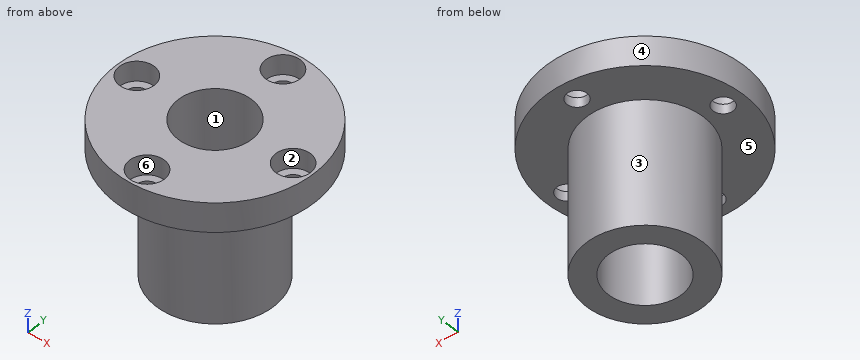
```python
from build123d import *

# Parameters (mm, degrees)
HOLE_WIZARD_1_D           = 5.5
HOLE_WIZARD_1_CBORE_D     = 9.5
HOLE_WIZARD_1_CBORE_DEPTH = 5.4


with BuildPart() as part:
    # 草图1 → 旋转1 (revolve)
    with BuildSketch(Plane(origin=(0, 0, 0), x_dir=(0, 0, 1), z_dir=(0, -1, 0))):
        Polygon((0, 10), (42, 10), (42, 27), (34, 27), (34, 16), (0, 16), align=None)
    revolve(axis=Axis((0, 0, 0), (0, 0, 1)))

    # 孔1 (through all)
    with Locations(Plane.XY.offset(42)):
        with Locations((0, -21.5), (-21.5, 0), (0, 21.5), (21.5, 0)):
            CounterBoreHole(HOLE_WIZARD_1_D / 2, HOLE_WIZARD_1_CBORE_D / 2, HOLE_WIZARD_1_CBORE_DEPTH)


solid = part.part
```
The listing builds one solid part. Answer for the finished solid, in the listing's coordinates (mm). Face numbers are marked on the shaded views. A direction names the side the tool comes from. Coordinates: 2 decimals unless noted, no trailing zeros. Write each loop counter-clockwise with the first axis right and the second up, starting at its lowest first coordinate (ties: lowest second). Pieces come first, ordered by that corner, then holes. Notation, with made-up numbers: M 3.5,-17.75 L 41.5,-17.75 A30 ccw 41.5,14.25 Z; hole C 46,75 d4. An arc over 180 degrees is marked long. Use a Markdown table: item, result. Add a question column.
1. For a pull along X with two mould halves and no side action, classify the marked faces 4, 5 and 6 as +X half, -X half, draft (parallel to the pull), parting line (faces both ways), or undercut.
2. Section C-C (z = 3) is taken. Give the vertices of the cut face in (x, y).
3. Straight lines are drawn through the part: line 1 along X through (y, z) = (0, 19); line 2 along Y through (x, z) = (0, 35.6); line 3 along Z through (x, y) = (16.5, 13). For each, find the intervals that lie inside material, in ascending order. Write a range as [from, to].
4. Which of the six approach directions +Z, -Z, +X, -X, +Y, -Y give full straight-line access (tool end or side, diameter ignored) to the marked faces 1, 2 and 3?
5. Given P1, Ø7.5, axis at x = 0, y = 23.5, coming from the +Z side; P2, Ø6.5, axis at x = 21.5, y = 0, coming from the -Z side; P3, Ø8, axis at x = -12, z = 14, coming from the -Y side; P4, Ø4, axis at x = -21, z = 33, coming from the -Y side, each flat-ended and moving along its own axis, determine where each tip first touches the part or whether it passes through.
6. Section A-A (y = 0) is taken. Give the vertices of the cut face in (x, z).
7. Section B-B (x = 21.5) is taken. Give the vertices of the cut face in (y, z).
Data:
| question | item | result |
|---|---|---|
| 1 | face 4 | parting line |
| 1 | face 5 | draft |
| 1 | face 6 | undercut |
| 2 | outline | C 0,0 d32; hole C 0,0 d20 |
| 3 | line 1 | x = [-16, -10], [10, 16] |
| 3 | line 2 | y = [-27, -24.25], [-18.75, -10], [10, 18.75], [24.25, 27] |
| 3 | line 3 | z = [34, 42] |
| 4 | face 1 | +Z, -Z |
| 4 | face 2 | +Z |
| 4 | face 3 | -Z |
| 5 | P1 | stops at z = 42 |
| 5 | P2 | stops at z = 34 |
| 5 | P3 | stops at y = -13.86 |
| 5 | P4 | stops at y = -18.91 |
| 6 | outline | M -27,34 L -24.25,34 L -24.25,36.6 L -26.25,36.6 L -26.25,42 L -27,42 Z; M -18.75,34 L -16,34 L -16,0 L -10,0 L -10,42 L -16.75,42 L -16.75,36.6 L -18.75,36.6 Z; M 10,0 L 16,0 L 16,34 L 18.75,34 L 18.75,36.6 L 16.75,36.6 L 16.75,42 L 10,42 Z; M 24.25,34 L 27,34 L 27,42 L 26.25,42 L 26.25,36.6 L 24.25,36.6 Z |
| 7 | outline | M -16.33,34 L -2.75,34 L -2.75,36.6 L -4.75,36.6 L -4.75,42 L -16.33,42 Z; M 2.75,34 L 16.33,34 L 16.33,42 L 4.75,42 L 4.75,36.6 L 2.75,36.6 Z |
